Check sheet for the modelled part. Datum: model origin and axes. Units: mm. Round coordinates to 2 decimals unless told otherwise and drop trailing zeros. Write each loop counter-clockwise with the first axis right and the second up, starting at its lowest first coordinate (ties: lowest second). Pieces come first, ordered by that corner, then holes. Notation, with made-up numbers: M 58.5,85 L 103.5,85 A20 cw 103.5,110 Z; hole C 72.5,24 d9. An arc over 180 degrees is marked long. One line per item, written item: value.
from build123d import *

# Parameters (mm, degrees)
SKETCH1_W           = 131
SKETCH1_H           = 30
BOSS_EXTRUDE1_DEPTH = 7
SKETCH2_R           = 2
CUT_EXTRUDE1_DEPTH  = 10


with BuildPart() as part:
    # Sketch1 → Boss-Extrude1 (new body)
    with BuildSketch(Plane(origin=(0, 0, 0), x_dir=(1, 0, 0), z_dir=(0, 1, 0))):
        with Locations((-37.010460251, 50.167364017)):
            Rectangle(SKETCH1_W, SKETCH1_H)
    extrude(amount=BOSS_EXTRUDE1_DEPTH)

    # Sketch2 → Cut-Extrude1 (cut)
    with BuildSketch(Plane.XZ):
        with Locations((-70.260460251, -61.167364017)):
            Circle(SKETCH2_R)
        with Locations((-41.010460251, -61.167364017)):
            Circle(SKETCH2_R)
        with Locations((-11.760460251, -61.167364017)):
            Circle(SKETCH2_R)
        with Locations((-11.760460251, -41.167364017)):
            Circle(SKETCH2_R)
        with Locations((-41.010460251, -41.167364017)):
            Circle(SKETCH2_R)
    extrude(amount=-CUT_EXTRUDE1_DEPTH, mode=Mode.SUBTRACT)


solid = part.part
Q1. Sectioned sample at A-A on y = 4. Enter the section's corners in (x, z).
Completed:
outline: M -102.51,-65.17 L 28.49,-65.17 L 28.49,-35.17 L -102.51,-35.17 Z; hole C -70.26,-61.17 d4; hole C -41.01,-61.17 d4; hole C -41.01,-41.17 d4; hole C -11.76,-61.17 d4; hole C -11.76,-41.17 d4
Q2. Scan lines: line 1 (X direction, y = 2.5, z = -42); line 2 (Z direction, x = -12.5, y = 4.5). Record each from-to range of solid material in increasing order. Write a range as [from, to].
Completed:
line 1: [-102.51, -42.83], [-39.19, -13.58], [-9.94, 28.49]
line 2: [-65.17, -63.03], [-59.31, -43.03], [-39.31, -35.17]
Q3. Depth check by flat-ended pin: P1, Ø3.5, axis at x = -11.76, z = -41.17, coming from the -Y side. Enter the tip coordinate at first touch or a pass-through.
Completed:
P1: through
Q4. Draft check along Z on faces 1 (the flat face through (-38, 7, -50)), 2 (the flat face through (-38, 3, -65.167)), 3 (the cylindrical face through (-10.838, 3.451, -42.942)), 4 (the flat face through (-38, 3, -35.167)). Enter one of: pulls with the +Z half, pulls with the -Z half, needs draft (parallel to the pull), parting line crosses it, or undercut.
Completed:
face 1: needs draft
face 2: pulls with the -Z half
face 3: undercut
face 4: pulls with the +Z half
